from build123d import *

# Parameters (mm, degrees)
F2_W     = 100.6348691881
F2_H     = 25.2255089581
F3_DEPTH = 25.4
F4_W     = 100.976370275
F4_H     = 23.4190355986
F5_DEPTH = 25.4
F8_W     = 101.243507117
F8_H     = 21.9049286097
F9_DEPTH = 25.4


# Not quite as in the source:
# - the program builds the solid bodies; features that only make, move or delete a surface that nothing else refers to are left out


with BuildPart() as f3:
    # F2 (on Top) → F3 (new body)
    with BuildSketch(Plane.XY):
        with Locations((-5.2274335176, -12.6127544791)):
            Rectangle(F2_W, F2_H)
    extrude(amount=F3_DEPTH)

    # F4 (on Front) → F5 (join)
    with BuildSketch(Plane.XZ):
        with Locations((-5.2071809769, -11.7095177993)):
            Rectangle(F4_W, F4_H)
    extrude(amount=F5_DEPTH)

    # F8 (on Front) → F9 (join)
    with BuildSketch(Plane.XZ):
        with Locations((-5.0736125559, -34.3714999035)):
            Rectangle(F8_W, F8_H)
    extrude(amount=F9_DEPTH)


solid = f3.part
Source: CAD feature listing. Evaluate the final solid. Frame: model axes, mm. A direction names the side the tool comes from. Give positions to 0.01 mm unless a question says otherwise; leave off trailing zeros. Return JSON: item names as keys, results as strings. Group by question number.
1) Material intervals for line 1 along Y through (x, z) = (-31, 20); line 2 along X through (y, z) = (-11, -8); line 3 along X through (y, z) = (-2.75, 7.5), sorted ascending. Write a range as [from, to].
2) Pin query (flat end, axial travel): P1, Ø10, axis at y = -22.5, z = -15.5, coming from the +X side; P2, Ø12.5, axis at y = -15, z = 9, coming from the -X side. Return the tip coordinate at first contact, or that it passes through.
3) Set-up query: faces 1 (the face through (-6, -25.226, 13)), 2 (the face through (45.281, -13, -12)), 3 (the face through (-55.545, -13, 13)). Return all of +Z, -Z, +X, -X, +Y, -Y with unobstructed straight access to the full face (end or side cutting, diameter ignored); none if empty.
Recorded:
{
 "1": {"line 1": "y = [-25.23, 0]", "line 2": "x = [-55.7, 45.28]", "line 3": "x = [-55.54, 45.09]"},
 "2": {"P1": "stops at x = 45.28", "P2": "stops at x = -55.54"},
 "3": {"face 1": "+Z, +X, -X, -Y", "face 2": "+Z, +X, +Y, -Y", "face 3": "+Z, -X, +Y, -Y"}
}
